Could you check a few things on this model? Use its own coordinates, in mm. Coordinates: 2 decimals unless noted, no trailing zeros. Write each loop counter-clockwise with the first axis right and the second up, starting at its lowest first coordinate (ties: lowest second). Pieces come first, ordered by that corner, then holes.
```python
from build123d import *

# Parameters (mm, degrees)
SKETCH_1_R          = 2.5
EXTRUDE_1_DEPTH     = 4
SKETCH_2_R          = 1.5
CUT_EXTRUDE_1_DEPTH = 4


with BuildPart() as part:
    # 草图1 → 凸台-拉伸1 (new body)
    with BuildSketch(Plane(origin=(0, 0, 0), x_dir=(1, 0, 0), z_dir=(0, 1, 0))):
        with BuildLine():
            Line((-125, 12), (125, 12))
            ThreePointArc((125, 12), (137, 0), (125, -12))
            Line((125, -12), (-125, -12))
            ThreePointArc((-125, -12), (-137, 0), (-125, 12))
        make_face()
        with Locations(Location((125, 0, 0), (0, 0, 270))):
            Circle(SKETCH_1_R, mode=Mode.SUBTRACT)
        with Locations(Location((-125, 0, 0), (0, 0, 270))):
            Circle(SKETCH_1_R, mode=Mode.SUBTRACT)
    extrude(amount=EXTRUDE_1_DEPTH)

    # 草图2 → 切除-拉伸1 (cut)
    with BuildSketch(Plane.XZ):
        with Locations(Location((-70, 0, 0), (0, 0, 270))):
            Circle(SKETCH_2_R)
        with Locations(Location((0, 0, 0), (0, 0, 270))):
            Circle(SKETCH_2_R)
        with Locations(Location((70, 0, 0), (0, 0, 270))):
            Circle(SKETCH_2_R)
    extrude(amount=-CUT_EXTRUDE_1_DEPTH, mode=Mode.SUBTRACT)


solid = part.part
```
Item 1: I want a section at A-A, the plane y = 3.3. List the corners of the cut face in (x, z) for me.
Item 2: Will these pins go through, and if not, where does the flat tip stop? pin 1 Ø4 at (x, z) = (70, 0) entering from -Y; pin 2 Ø1.5 at (y, z) = (0.5, 6) entering from -X.
Item 3: If I drill on line 1 along X through (y, z) = (2.65, 0); line 2 along Z through (x, y) = (-70, 2.85); line 3 along X through (y, z) = (1.3, 6.25), over which ranges is the centre line in solid material (lowest first)?
Item 4: I want a section at B-B, the plane z = 8.5. List the corners of the cut face in (x, y) for me.
Item 5: If we mould it in two halves opening along X, with no side actions, what happens to faces 1 (the cylindrical face through (-122.52, 1.97, -0.33)), 2 (the cylindrical face through (-137, 2, 0)), 3 (the cylindrical face through (127.48, 1.97, -0.33)), 4 (the cylindrical face through (137, 2, 0))? For each: released by +X, released by -X, zero draft, split by the parting line, or undercut.
Item 6: I want a section at C-C, the plane z = -9. List the corners of the cut face in (x, y) for me, then the cut area to 3 significant figures.
Taken from the geometry:
1. outline: (-125, -12) - (125, -12) arc R12 ccw to (125, 12) - (-125, 12) arc R12 ccw to start; hole circle Ø5 at (-125, 0); hole circle Ø3 at (-70, 0); hole circle Ø3 at (0, 0); hole circle Ø3 at (70, 0); hole circle Ø5 at (125, 0)
2. pin 1: stops at y = 0
2. pin 2: stops at x = -135.79
3. line 1: x = -137 to -127.5, -122.5 to -71.5, -68.5 to -1.5, 1.5 to 68.5, 71.5 to 122.5, 127.5 to 137
3. line 2: z = -12 to -1.5, 1.5 to 12
3. line 3: x = -135.24 to 135.24
4. outline: (-133.47, 0) - (133.47, 0) - (133.47, 4) - (-133.47, 4) - close
5. face 1: undercut
5. face 2: released by -X
5. face 3: undercut
5. face 4: released by +X
6. outline: (-132.94, 0) - (132.94, 0) - (132.94, 4) - (-132.94, 4) - close
6. area: 1,060 mm2
